from build123d import *

# Parameters (mm, degrees)
SKETCH4_W           = 200
SKETCH4_H           = 180
BOSS_EXTRUDE3_DEPTH = 2
SKETCH4_3_W         = 204
SKETCH4_3_H         = 184
SKETCH4_3_W_2       = 200
SKETCH4_3_H_2       = 180
BOSS_EXTRUDE4_DEPTH = 42
SKETCH6_R           = 2
BOSS_EXTRUDE5_DEPTH = 40
SKETCH8_R           = 1
CUT_EXTRUDE1_DEPTH  = 40
SKETCH5_R           = 2
SKETCH5_W           = 15
SKETCH5_H           = 20
SKETCH5_W_2         = 21
SKETCH5_H_2         = 15
CUT_EXTRUDE2_DEPTH  = 2


with BuildPart() as part:
    # Sketch4 → Boss-Extrude3 (new body)
    with BuildSketch(Plane(origin=(0, 0, 0), x_dir=(1, 0, 0), z_dir=(0, 1, 0))):
        Rectangle(SKETCH4_W, SKETCH4_H)
    extrude(amount=BOSS_EXTRUDE3_DEPTH)

    # Sketch4_3 → Boss-Extrude4 (add)
    with BuildSketch(Plane(origin=(0, 0, 0), x_dir=(1, 0, 0), z_dir=(0, 1, 0))):
        Rectangle(SKETCH4_3_W, SKETCH4_3_H)
        Rectangle(SKETCH4_3_W_2, SKETCH4_3_H_2, mode=Mode.SUBTRACT)
    extrude(amount=BOSS_EXTRUDE4_DEPTH)

    # Sketch6 → Boss-Extrude5 (add)
    with BuildSketch(Plane(origin=(0, 2, 0), x_dir=(1, 0, 0), z_dir=(0, 1, 0))):
        with Locations(Location((-5, -80, 0), (0, 0, 90))):
            Circle(SKETCH6_R)
        with Locations(Location((-5, 80, 0), (0, 0, 90))):
            Circle(SKETCH6_R)
        with Locations(Location((85, -20, 0), (0, 0, 90))):
            Circle(SKETCH6_R)
        with Locations(Location((-85, 20, 0), (0, 0, 90))):
            Circle(SKETCH6_R)
    extrude(amount=BOSS_EXTRUDE5_DEPTH)

    # Sketch8 → Cut-Extrude1 (cut)
    with BuildSketch(Plane(origin=(0, 42, 0), x_dir=(1, 0, 0), z_dir=(0, 1, 0))):
        with Locations(Location((-5, 80, 0), (0, 0, 270))):
            Circle(SKETCH8_R)
        with Locations(Location((85, -20, 0), (0, 0, 270))):
            Circle(SKETCH8_R)
        with Locations(Location((-5, -80, 0), (0, 0, 270))):
            Circle(SKETCH8_R)
        with Locations(Location((-85, 20, 0), (0, 0, 270))):
            Circle(SKETCH8_R)
    extrude(amount=-CUT_EXTRUDE1_DEPTH, mode=Mode.SUBTRACT)

    # Sketch5 → Cut-Extrude2 (cut)
    with BuildSketch(Plane(origin=(0, 0, -92), x_dir=(-1, 0, 0), z_dir=(0, 0, -1))):
        with Locations((58.311430335, 24.978671474)):
            Circle(SKETCH5_R)
        with Locations((31.311430335, 24.978671474)):
            Circle(SKETCH5_R)
        with Locations((84.5, 23.893749762)):
            Rectangle(SKETCH5_W, SKETCH5_H)
        with Locations((44.811430335, 24.978671474)):
            Rectangle(SKETCH5_W_2, SKETCH5_H_2)
    extrude(amount=-CUT_EXTRUDE2_DEPTH, mode=Mode.SUBTRACT)


solid = part.part
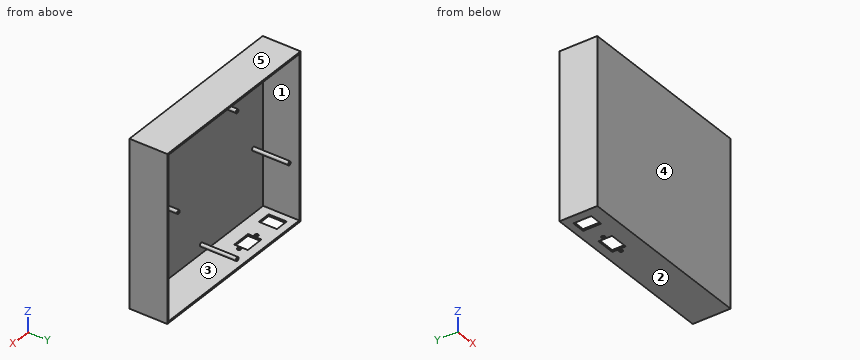
For this review, take the finished solid that the model builds, in its own axes (mm). Face numbers are marked on the shaded views. A direction names the side the tool comes from. Coordinates: 2 decimals unless noted, no trailing zeros. Loops run counter-clockwise (first coordinate to the right, second up) from the corner with the lowest first, then second, coordinate; pieces in that order, holes last. Notation, with made-up numbers: (-8.5, 15.5) -> (-1.5, 15.5) arc R21 ccw to (-1.5, 51.5) -> close; hole circle Ø2 at (-31.75, 74.25). An arc over 180 degrees is marked (long way). Write each question's results on one line, items separated by ' | '.
Q1. To check wall thickness, follow line 1 along X through (y, z) = (3, -20); line 2 along X through (y, z) = (16, 80); line 3 along X through (y, z) = (20, -4.5). State the ranges of each line that lie inside material, in increasing order. Write a range as [from, to].
Taken from the geometry:
line 1: [-102, -100], [-87, -86], [-84, -83], [100, 102] | line 2: [-102, -100], [-7, -6], [-4, -3], [100, 102] | line 3: [-102, -100], [100, 102]
Q2. Machinability: for the marked faces 1 and 2, which of the approach directions +Z, -Z, +X, -X, +Y, -Y give a long, thin tool a straight path to every point of the face, cutting with its end or side? Answer none if there is none.
Taken from the geometry:
face 1: +Y | face 2: -Z, +X, -X, +Y, -Y
Q3. For pin 1 Ø0.6 at (x, z) = (85, 20) entering from +Y, flat-tipped, find the tip position at first contact; note if it passes through.
Taken from the geometry:
pin 1: y = 2
Q4. Add section A-A, the plane y = 20. Count the separate pieces of the cut face and the enclosed holes in it, then the cut area to 3 significant figures.
Taken from the geometry:
separate pieces: 6 | enclosed holes: 4 | area: 1,500 mm²
Q5. Add section B-B, the plane x = -64.5. State the section outline as (y, z) points.
Taken from the geometry:
outline: (0, -92) -> (42, -92) -> (42, -90) -> (2, -90) -> (2, 90) -> (42, 90) -> (42, 92) -> (0, 92) -> close
Q6. Mouldability with a two-part tool opening along Z and no side actions: class the marked faces 3, 4 and 5 as +Z half, -Z half, draft (parallel to the pull), parting line (faces both ways), or undercut.
Taken from the geometry:
face 3: undercut | face 4: draft | face 5: +Z half
Q7. Add section C-C, the plane z = -5.5. State the section outline as (x, y) points, then the cut area to 3 significant figures.
Taken from the geometry:
outline: (-102, 0) -> (102, 0) -> (102, 42) -> (100, 42) -> (100, 2) -> (-100, 2) -> (-100, 42) -> (-102, 42) -> close | area: 568 mm²
